Verification items for the finished model (mm, model axes). A direction names the side the tool comes from. Coordinates: 2 decimals unless noted, no trailing zeros. Loops run counter-clockwise (first coordinate to the right, second up) from the corner with the lowest first, then second, coordinate; pieces in that order, holes last. Notation, with made-up numbers: (10, -29.5) -> (49, -29.5) arc R16 cw to (49, -11.5) -> close; hole circle Ø6 at (2, -10). An arc over 180 degrees is marked (long way). Write item = value, one per line.
```python
from build123d import *

# Parameters (mm, degrees)
F0_W     = 692
F0_H     = 12
F1_DEPTH = 65
F2_W     = 5
F2_H     = 5
F3_DEPTH = 709
F4_W     = 5
F4_H     = 4.429847
F5_DEPTH = 709
F6_W     = 5
F6_H     = 5
F7_DEPTH = 509
F8_W     = 5
F8_H     = 492
F9_DEPTH = 12


with BuildPart() as f1:
    # F0 (on Front) → F1 (new body)
    with BuildSketch(Plane.XZ):
        Polygon((59.521648, 466.902112), (-632.478352, 466.902112), (-636.478352, 466.902112), (-636.478352, 454.902112), (-632.478352, 454.902112), (59.521648, 454.902112), (63.521648, 454.902112), (63.521648, 466.902112), align=None)
        Polygon((-634.478352, 630.902112), (-644.478352, 630.902112), (-644.478352, -49.097888), (-632.478352, -49.097888), (-632.478352, -37.097888), (-632.478352, 454.902112), (-636.478352, 454.902112), (-636.478352, 466.902112), (-632.478352, 466.902112), (-632.478352, 618.902112), (-632.478352, 630.902112), align=None)
        with Locations((-286.478352, 624.902112)):
            Rectangle(F0_W, F0_H)
        Polygon((71.521648, 630.902112), (59.521648, 630.902112), (59.521648, 618.902112), (59.521648, 466.902112), (63.521648, 466.902112), (63.521648, 454.902112), (59.521648, 454.902112), (59.521648, -37.097888), (59.521648, -49.097888), (71.521648, -49.097888), align=None)
        with Locations((-286.478352, -43.097888)):
            Rectangle(F0_W, F0_H)
    extrude(amount=F1_DEPTH)

    # F2 (on face) → F3 (cut)
    with BuildSketch(Plane.YZ.offset(71.521648)):
        with Locations((-56.5, -39.597888)):
            Rectangle(F2_W, F2_H)
    extrude(amount=-F3_DEPTH, mode=Mode.SUBTRACT)

    # F4 (on face) → F5 (cut)
    with BuildSketch(Plane.YZ.offset(71.521648)):
        with Locations((-56.5, 457.117035)):
            Rectangle(F4_W, F4_H)
    extrude(amount=-F5_DEPTH, mode=Mode.SUBTRACT)

    # F6 (on face) → F7 (cut)
    with BuildSketch(Plane(origin=(0, 0, -49.097888), x_dir=(1, 0, 0), z_dir=(0, 0, -1))):
        with Locations((-634.978352, 56.5)):
            Rectangle(F6_W, F6_H)
    extrude(amount=-F7_DEPTH, mode=Mode.SUBTRACT)

    # F8 (on face) → F9 (cut)
    with BuildSketch(Plane.YZ.offset(71.521648)):
        with Locations((-56.5, 208.902112)):
            Rectangle(F8_W, F8_H)
    extrude(amount=-F9_DEPTH, mode=Mode.SUBTRACT)


solid = f1.part
```
1) Release check for a two-part mould opening along Y. For faces 1 (the face through (-124, -59, -41)), 2 (the face through (-291, -32, 618.902)), 3 (the face through (-447, 0, 620)) record: pulls with the +Y half, pulls with the -Y half, needs draft (parallel to the pull), parting line crosses it, or undercut.
Ans:
face_1 = undercut
face_2 = needs draft
face_3 = pulls with the +Y half
2) Sectioned sample at A-A, the plane z = 287. Record the cut outline in (x, y).
Ans:
outline = (-644.48, -65) -> (-632.48, -65) -> (-632.48, -59) -> (-637.48, -59) -> (-637.48, -54) -> (-632.48, -54) -> (-632.48, 0) -> (-644.48, 0) -> close; (59.52, -65) -> (71.52, -65) -> (71.52, -59) -> (59.52, -59) -> close; (59.52, -54) -> (71.52, -54) -> (71.52, 0) -> (59.52, 0) -> close
3) Depth check by flat-ended pin: pin 1 Ø1.5 at (x, y) = (-635.5, -56.5) entering from -Z. Enter the tip coordinate at first touch or a pass-through.
Ans:
pin_1 = 459.9
4) Sectioned sample at C-C, the plane y = -36. Record the cut outline in (x, z).
Ans:
outline = (-644.48, -49.1) -> (71.52, -49.1) -> (71.52, 630.9) -> (-644.48, 630.9) -> close; hole (-632.48, -37.1) -> (59.52, -37.1) -> (59.52, 454.9) -> (-632.48, 454.9) -> close; hole (-632.48, 466.9) -> (59.52, 466.9) -> (59.52, 618.9) -> (-632.48, 618.9) -> close
5) Material ranges on line 1 (Z direction, x = -247, y = -14.5); line 2 (Z direction, x = -0.5, y = -55.5); line 3 (X direction, y = -33, z = 185.5), recorded low to high.
Ans:
line_1 = -49.1 to -37.1, 454.9 to 466.9, 618.9 to 630.9
line_2 = -49.1 to -42.1, 459.33 to 466.9, 618.9 to 630.9
line_3 = -644.48 to -632.48, 59.52 to 71.52
6) Tool access check on faces 4 (the face through (-281, -32, 630.902)), 5 (the face through (59.522, -32, 544)). Record the directions out of +Z, -Z, +X, -X, +Y, -Y that give a thin tool (end or side, any length) a straight path to the whole face; none if there is none.
Ans:
face_4 = +Z, +X, -X, +Y, -Y
face_5 = +Y, -Y
7) Sectioned sample at B-B, the plane x = -102.5. Record the cut outline in (y, z), plus the area to 3 significant figures.
Ans:
outline = (-65, -49.1) -> (0, -49.1) -> (0, -37.1) -> (-54, -37.1) -> (-54, -42.1) -> (-59, -42.1) -> (-59, -37.1) -> (-65, -37.1) -> close; (-65, 454.9) -> (-59, 454.9) -> (-59, 459.33) -> (-54, 459.33) -> (-54, 454.9) -> (0, 454.9) -> (0, 466.9) -> (-65, 466.9) -> close; (-65, 618.9) -> (0, 618.9) -> (0, 630.9) -> (-65, 630.9) -> close
area = 2,290 mm2
